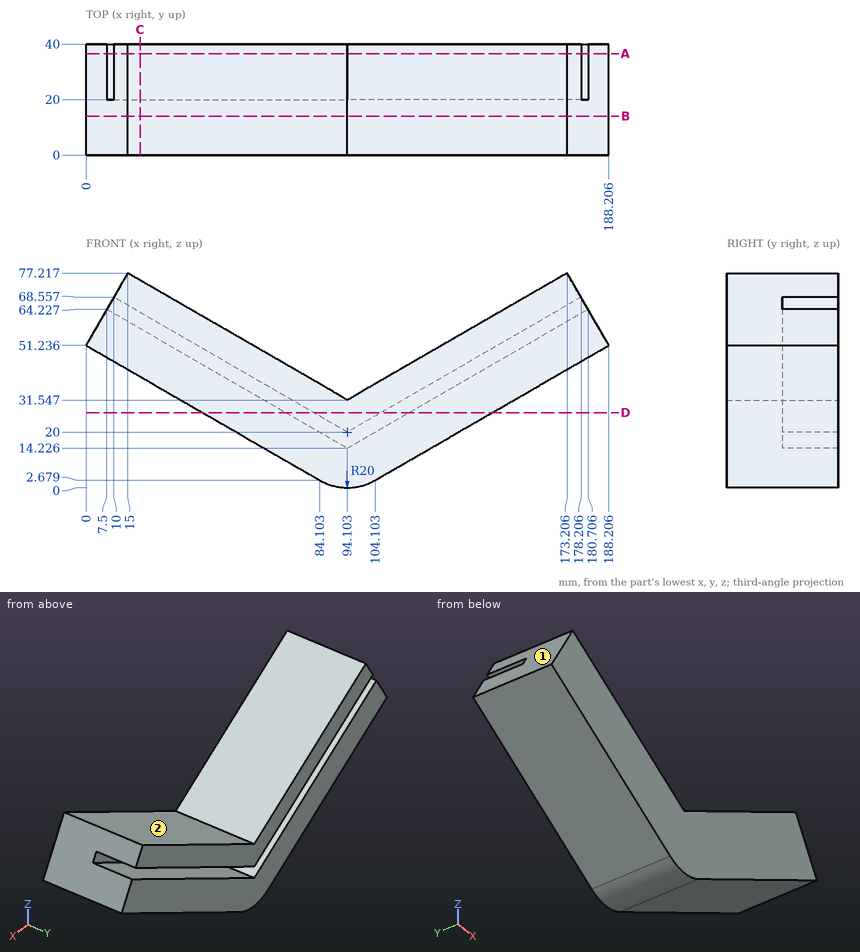
Here's the drawing with two shaded views (mm, measured from the low corner). I have some questions. A direction names the side the tool comes from. Coordinates: 2 decimals unless noted, no trailing zeros. Order: outer loops, then holes, each group sorted by start corner. A loop starts at its lowest first (then second) coordinate and runs counter-clockwise, first axis right, second up. Notation, with made-up numbers: (1, -3) - (31, -3) arc R27 ccw to (31, 23) - close; hole circle Ø10 at (53, 38.25). An arc over 180 degrees is marked (long way). Answer in a Markdown table with one row per item.
1. For the marked faces 1 and 2, which set-ups out of +Z, -Z, +X, -X, +Y, -Y let a thin tool reach every point of the face, with its end or its side?
Reply:
| item | result |
|---|---|
| face 1 | +Z, -X, +Y, -Y |
| face 2 | +Z, +Y, -Y |
2. Suppose I cut it at D-D (z = 27). Please give me the cut outline in (x, y).
Reply:
| item | result |
|---|---|
| outline | (41.98, 0) - (146.23, 0) - (146.23, 40) - (116.23, 40) - (116.23, 20) - (106.23, 20) - (106.23, 40) - (81.98, 40) - (81.98, 20) - (71.98, 20) - (71.98, 40) - (41.98, 40) - close |
3. Suppose I cut it at C-C (x = 19.5). Please give me the cut outline in (y, z), and give its area (3 significant figures).
Reply:
| item | result |
|---|---|
| outline | (0, 39.98) - (40, 39.98) - (40, 57.3) - (20, 57.3) - (20, 63.07) - (40, 63.07) - (40, 74.62) - (0, 74.62) - close |
| area | 1,270 mm^2 |
4. Suppose I cut it at B-B (y = 14). Please give me the cut outline in (x, z) (1 decimal).
Reply:
| item | result |
|---|---|
| outline | (0, 51.2) - (84.1, 2.7) arc R20 ccw to (104.1, 2.7) - (188.2, 51.2) - (173.2, 77.2) - (94.1, 31.5) - (15, 77.2) - close |
5. If I drill on line 1 along X through (y, z) = (27, 56.5) (1 decimal); line 2 along Z through (x, y) = (129.5, 26.5) (1 decimal); line 3 along Z through (x, y) = (78, 31.5) (1 decimal), over which ranges is the centre line in solid material (lowest first)?
Reply:
| item | result |
|---|---|
| line 1 | x = 3 to 20.9, 30.9 to 50.9, 137.3 to 157.3, 167.3 to 185.2 |
| line 2 | z = 17.3 to 34.7, 40.4 to 52 |
| line 3 | z = 6.2 to 23.5, 29.3 to 40.8 |
6. For pin 1 (5 mm diameter, centred on x = 75, y = 28.5, fed in from -Z); pin 2 (1 mm diameter, centred on x = 118, y = 30.5, fed in from +Z); pin 3 (12 mm diameter, centred on y = 9.5, z = 44, fed in from +X) (1 decimal), each with a flat end and sliding along its axis, tell me the tip position at first contact or that it passes through.
Reply:
| item | result |
|---|---|
| pin 1 | stops at z = 6.49 |
| pin 2 | stops at z = 45.63 |
| pin 3 | stops at x = 186.1 |
7. Suppose I cut it at A-A (y = 36.5). Please give me the cut outline in (x, z) (1 decimal), and give its area (3 significant figures).
Reply:
| item | result |
|---|---|
| outline | (0, 51.2) - (84.1, 2.7) arc R20 ccw to (104.1, 2.7) - (188.2, 51.2) - (180.7, 64.2) - (94.1, 14.2) - (7.5, 64.2) - close; (10, 68.6) - (94.1, 20) - (178.2, 68.6) - (173.2, 77.2) - (94.1, 31.5) - (15, 77.2) - close |
| area | 4,990 mm^2 |
